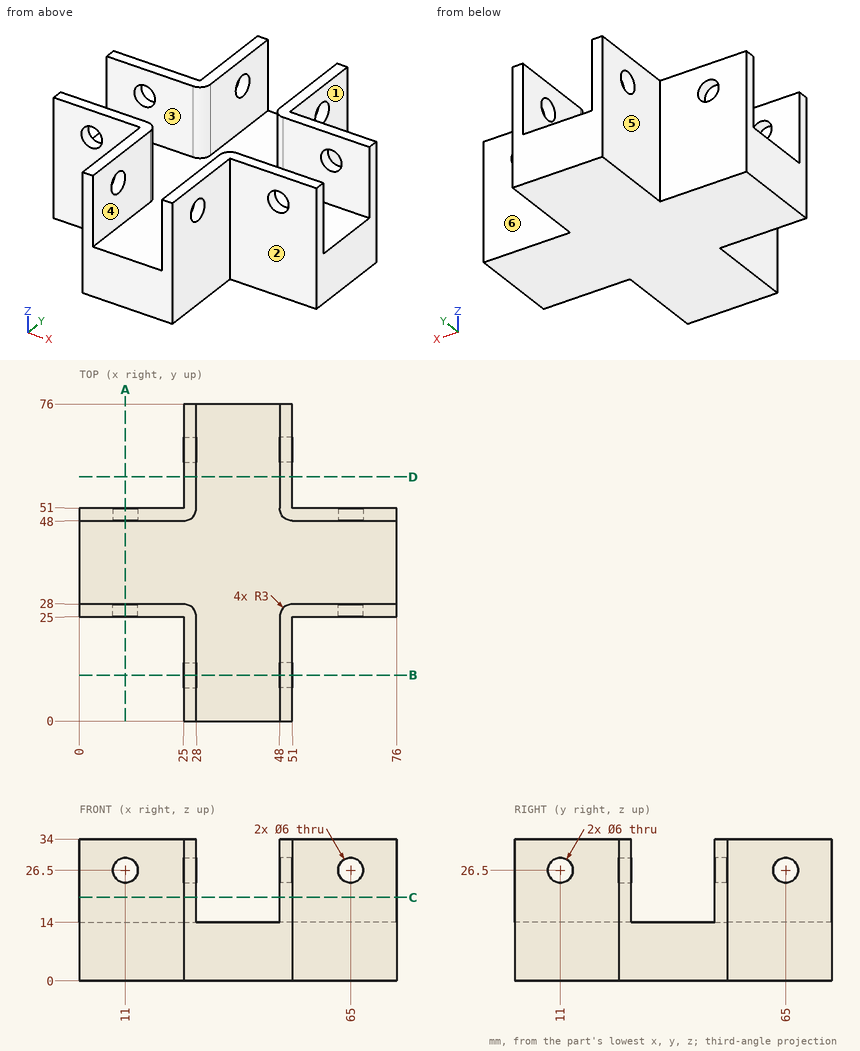
Here's the drawing with two shaded views (mm, measured from the low corner). I have some questions. A direction names the side the tool comes from. Round coordinates to 2 decimals unless told otherwise and drop trailing zeros. Order: outer loops, then holes, each group sorted by start corner. A loop starts at its lowest first (then second) coordinate and runs counter-clockwise, first axis right, second up. Notation, with made-up numbers: (-36.75, 86.5) -> (-28.75, 86.5) arc R17 ccw to (-28.75, 94.5) -> close; hole circle Ø2 at (-5.75, 66). An arc over 180 degrees is marked (long way). Use a Markdown table: item, result. Add a question column.
(1) I need wall thicknesses on line 1 along Y through (x, z) = (27, 26); line 2 along Y through (x, z) = (59.5, 25.5). Which ranges of each line are inside material? Lowest first, please.
(2) Suppose I cut it at D-D, the plane y = 58.5. Please give me the cut outline in (x, z).
(3) If we mould it in two halves opening along Y, with no side actions, what happens to the marked faces 1, 2 and 3? For each: released by +Y, released by -Y, zero draft, split by the parting line, or undercut.
(4) For pin 1 Ø6 at (x, y) = (41, 51) entering from -Z; pin 2 Ø6 at (y, z) = (17.5, 26.5) entering from +X; pin 3 Ø7.5 at (x, z) = (66, 16.5) entering from -Y; pin 4 Ø20 at (y, z) = (8, 10.5) entering from -X, each with a flat end and sliding along its axis, tell me the tip position at first contact or that it passes through.
(5) Suppose I cut it at C-C, the plane z = 20. Please give me the cut outline in (x, y).
(6) Suppose I cut it at A-A, the plane x = 11. Please give me the cut outline in (y, z).
(7) For the marked faces 4, 5 and 6, which set-ups out of +Z, -Z, +X, -X, +Y, -Y let a thin tool reach every point of the face, with its end or its side?
Verdict:
| question | item | result |
|---|---|---|
| 1 | line 1 | 0 to 8.04, 13.96 to 27.24, 48.76 to 62.04, 67.96 to 76 |
| 1 | line 2 | 25 to 28, 48 to 51 |
| 2 | outline | (25, 0) -> (51, 0) -> (51, 34) -> (48, 34) -> (48, 14) -> (28, 14) -> (28, 34) -> (25, 34) -> close |
| 3 | face 1 | zero draft |
| 3 | face 2 | released by -Y |
| 3 | face 3 | undercut |
| 4 | pin 1 | z = 0 |
| 4 | pin 2 | x = 51 |
| 4 | pin 3 | y = 25 |
| 4 | pin 4 | x = 25 |
| 5 | outline | (0, 25) -> (25, 25) -> (25, 0) -> (28, 0) -> (28, 25) arc R3 ccw to (25, 28) -> (0, 28) -> close; (0, 48) -> (25, 48) arc R3 ccw to (28, 51) -> (28, 76) -> (25, 76) -> (25, 51) -> (0, 51) -> close; (48, 0) -> (51, 0) -> (51, 25) -> (76, 25) -> (76, 28) -> (51, 28) arc R3 ccw to (48, 25) -> close; (48, 51) arc R3 ccw to (51, 48) -> (76, 48) -> (76, 51) -> (51, 51) -> (51, 76) -> (48, 76) -> close |
| 6 | outline | (25, 0) -> (51, 0) -> (51, 23.5) -> (48, 23.5) -> (48, 14) -> (28, 14) -> (28, 23.5) -> (25, 23.5) -> close; (25, 29.5) -> (28, 29.5) -> (28, 34) -> (25, 34) -> close; (48, 29.5) -> (51, 29.5) -> (51, 34) -> (48, 34) -> close |
| 7 | face 4 | +Z, +Y, -Y |
| 7 | face 5 | +Z, -Z, -X, +Y |
| 7 | face 6 | +Z, -Z, +X, +Y |
